Check sheet for the modelled part. Datum: model origin and axes. Units: mm. A direction names the side the tool comes from. Give positions to 0.01 mm unless a question says otherwise; leave off trailing zeros. Loops run counter-clockwise (first coordinate to the right, second up) from the corner with the lowest first, then second, coordinate; pieces in that order, holes last. Notation, with made-up numbers: M 67.25,-12.75 L 115.25,-12.75 A27 cw 115.25,10.25 Z; hole C 20,-40 d3. An arc over 180 degrees is marked long. Write each question's results on one line, items separated by ' | '. Start each with the question number.
1. Draft check along X on faces 3 (the flat face through (-4, 0, 0)), 4 (the flat face through (2.838, 0, 5)), 5 (the cylindrical face through (-7.39, -3.06, 20.27)), 6 (the flat face through (0, 0, 11)). Enter one of: pulls with the +X half, pulls with the -X half, needs draft (parallel to the pull), parting line crosses it, or undercut.
2. Sectioned sample at C-C on z = 31. Record the cut outline in (x, y).
3. Sectioned sample at A-A on y = 0. Record the cut outline in (x, z).
4. Go/stop test with flat-tipped pins: pin 1 (1.5 mm diameter, centred on x = 3.5, z = 22.5, fed in from -Y); pin 2 (6 mm diameter, centred on y = 5, z = 15.5, fed in from -X). Record where each tip stops, or that it passes through.
5. Sectioned sample at B-B on x = 0. Record the cut outline in (y, z), and give its area (3 significant figures).
6. Tool access check on faces 1 (the conical face through (7.2, 0.1, 0.2)), 2 (the flat face through (-2.662, 0, 5)). Record the directions out of +Z, -Z, +X, -X, +Y, -Y that give a thin tool (end or side, any length) a straight path to the whole face; none if there is none.
7. Material ranges on line 1 along X through (y, z) = (7, 2); line 2 along Z through (x, y) = (0.5, 0); line 3 along X through (y, z) = (-0.25, 29), recorded low to high.
```python
from build123d import *

# Parameters (mm, degrees)
F0_W     = 8
F0_H     = 40
F2_W     = 5.5
F2_H     = 11
F3_DEPTH = 12.5
F4_SIZE  = 1


with BuildPart() as f1:
    # F0 (on Front) → F1 (revolve)
    with BuildSketch(Plane.XZ):
        with Locations((-4, 20)):
            Rectangle(F0_W, F0_H)
    revolve(axis=Axis((0, 0, 20), (0, 0, -1)))

    # F2 (on Front) → F3 (cut, symmetric)
    with BuildSketch(Plane.XZ):
        with Locations((0.0883303039, 5.5)):
            Rectangle(F2_W, F2_H)
    extrude(amount=F3_DEPTH, both=True, mode=Mode.SUBTRACT)

    # F4
    f4_edges = [f1.edges().sort_by_distance(p)[0] for p in [
        (8, 0, 40),
        (8, 0, 0),
        (-6.530442, 4.620965, 0),
        (-6.530442, -4.620965, 0),
    ]]
    chamfer(f4_edges, length=F4_SIZE)


solid = f1.part
```
Output values:
1) face 3: needs draft | face 4: undercut | face 5: parting line crosses it | face 6: undercut
2) outline: C 0,0 d16
3) outline: M -8,1 L -7,0 L -2.66,0 L -2.66,11 L 2.84,11 L 2.84,0 L 7,0 L 8,1 L 8,39 L 7,40 L -7,40 L -8,39 Z
4) pin 1: y = -7.51 | pin 2: x = -7.75
5) outline: M -8,11 L 8,11 L 8,39 L 7,40 L -7,40 L -8,39 Z | area: 463 mm2
6) face 1: -Z, +X | face 2: -Z, +Y, -Y
7) line 1: -3.87 to -2.66, 2.84 to 3.87 | line 2: 11 to 40 | line 3: -8 to 8
